```python
from build123d import *

# Parameters (mm, degrees)
SKETCH2_W          = 7
SKETCH2_H          = 1
SKETCH3_R          = 3.05
CUT_EXTRUDE1_DEPTH = 57.789083458
CHAMFER1_SIZE      = 2
SKETCH4_R          = 9
CUT_EXTRUDE2_DEPTH = 57.648036153


with BuildPart() as part:
    # Sketch2 → Revolve1 (revolve)
    with BuildSketch(Plane(origin=(0, 0, 0), x_dir=(1, 0, 0), z_dir=(0, 1, 0))):
        with Locations((3.5, -2.5)):
            Rectangle(SKETCH2_W, SKETCH2_H)
        with BuildLine():
            Line((0, 2), (0, -2))
            Line((0, -2), (7, -2))
            Line((7, -2), (7, -1))
            Line((7, -1), (35.767949192, -1))
            Line((35.767949192, -1), (37.5, -2))
            Line((37.5, -2), (40, -2))
            Line((40, -2), (40, -1))
            ThreePointArc((40, -1), (39, 0), (40, 1))
            Line((40, 1), (40, 2))
            Line((40, 2), (0, 2))
        make_face()
    revolve(axis=Axis((0, 0, 2), (0, 0, -1)))

    # Sketch3 → Cut-Extrude1 (cut, through all)
    with BuildSketch(Plane.XY.offset(3)):
        Circle(SKETCH3_R)
    extrude(amount=-CUT_EXTRUDE1_DEPTH, mode=Mode.SUBTRACT)

    # Chamfer1
    chamfer1_edges = [part.edges().sort_by_distance(p)[0] for p in [
        (-7, 0, 1),
    ]]
    chamfer(chamfer1_edges, length=CHAMFER1_SIZE - 0.0001)  # a hair under: the kernel refuses the full size

    # Sketch4 → Cut-Extrude2 (cut, through all)
    with BuildSketch(Plane.XY.offset(1)):
        with Locations((0, -22)):
            Circle(SKETCH4_R)
        with Locations((-20.923243358, -6.798373876)):
            Circle(SKETCH4_R)
        with Locations((-12.93127555, 17.798373876)):
            Circle(SKETCH4_R)
        with Locations((12.93127555, 17.798373876)):
            Circle(SKETCH4_R)
        with Locations((20.923243358, -6.798373876)):
            Circle(SKETCH4_R)
    extrude(amount=-CUT_EXTRUDE2_DEPTH, mode=Mode.SUBTRACT)


solid = part.part
```
Here's how the part is built. I have some questions about the finished solid (model axes, mm). A direction names the side the tool comes from. Coordinates: 2 decimals unless noted, no trailing zeros. Return JSON: item names as keys, results as strings. Group by question number.
Item 1: We'd pull the mould along Y, two halves only. Please class faces 3 (the face through (-14.103, 26.722, -0.479)), 4 (the face through (-8.67, 39.05, -1.51)), 5 (the face through (-12, -36, 2)): +Y half, -Y half, draft (parallel to the pull), parting line (faces both ways), or undercut.
Item 2: On a 3-axis mill with a long thin cutter (end or side, diameter ignored), from which of +Z, -Z, +X, -X, +Y, -Y can I reach the whole of each face in a straight line? I mean faces 1 (the face through (-7, 7, 1)), 2 (the face through (-1, 8, -2)). Say none if no direction works.
Item 3: If we section it at A-A on x = 0: State how many separate pieces and enclosed holes the cut face has, and give its area (3 significant figures).
Item 4: I need wall thicknesses on line 1 (Y direction, x = 0, z = -0.75); line 2 (Y direction, x = 20.5, z = 0.8); line 3 (Y direction, x = 0, z = 1.45). Which ranges of each line are inside material? Lowest first, please. Write a range as from..to.
Item 5: Will these pins go through, and if not, where does the flat tip stop? P1, Ø20.5, axis at x = 12.93, y = 17.8, coming from the +Z side; P2, Ø3, axis at x = -24.5, z = -0.5, coming from the -Y side; P3, Ø3, axis at x = -16.5, z = 1.5, coming from the -Y side; P4, Ø16, axis at x = 20.92, y = -6.8, coming from the -Z side.
Calculated:
{
 "1": {"face 3": "undercut", "face 4": "parting line", "face 5": "draft"},
 "2": {"face 1": "+Z", "face 2": "-Z, +X, -X, +Y, -Y"},
 "3": {"separate pieces": "3", "enclosed holes": "0", "area": "191 mm^2"},
 "4": {"line 1": "y = -39.34..-31, -13..-3.05, 3.05..39.34", "line 2": "y = -33.65..-15.79, 2.19..12.93, 22.67..33.65", "line 3": "y = -40..-36.55, -8.55..-3.05, 3.05..8.55, 36.55..40"},
 "5": {"P1": "stops at z = 1", "P2": "stops at y = -32.67", "P3": "stops at y = -37.08", "P4": "passes through"}
}
